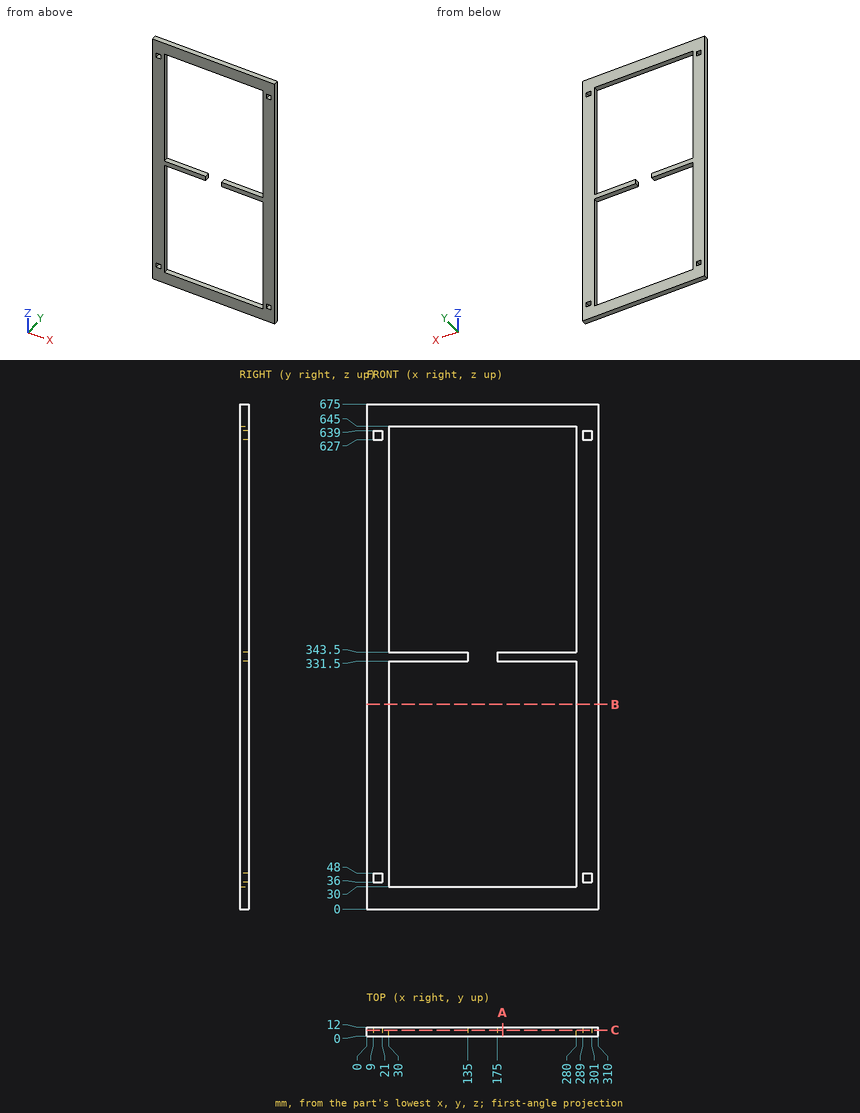
Study the drawing (mm; zero at the part's minimum x, y, z) and answer. Give positions to 0.01 mm unless a question says otherwise; leave off trailing zeros. Loops run counter-clockwise (first coordinate to the right, second up) from the corner with the lowest first, then second, coordinate; pieces in that order, holes last. Notation, with made-up numbers: (55, -9.75) - (110, -9.75) arc R11 cw to (110, -5.75) - close; hole circle Ø2 at (30, 7.25). An arc over 180 degrees is marked (long way). Return JSON: item names as keys, results as strings. Group by question number.
1. Find section C-C (y = 7.75). State how many separate pieces and enclosed holes the cut face has, then the cut area to 3 significant figures.
2. Find section B-B (z = 273.5). Write down the section's boundary in (x, y).
3. Find section A-A (x = 182). Write down the section's boundary in (y, z), then the cut area to 3 significant figures.
4. Straight lines are drawn through the part: line 1 (Z direction, x = 106, y = 11.25); line 2 (X direction, y = 8.5, z = 381); line 3 (Z direction, x = 142.5, y = 4.5). For each, find the intervals that lie inside material, in ascending order. Write a range as [from, to].
Verdict:
{
 "1": {"separate pieces": "1", "enclosed holes": "5", "area": "57,400 mm^2"},
 "2": {"outline": "(0, 0) - (30, 0) - (30, 12) - (0, 12) - close; (280, 0) - (310, 0) - (310, 12) - (280, 12) - close"},
 "3": {"outline": "(0, 0) - (12, 0) - (12, 30) - (0, 30) - close; (0, 331.5) - (12, 331.5) - (12, 343.5) - (0, 343.5) - close; (0, 645) - (12, 645) - (12, 675) - (0, 675) - close", "area": "864 mm^2"},
 "4": {"line 1": "z = [0, 30], [331.5, 343.5], [645, 675]", "line 2": "x = [0, 30], [280, 310]", "line 3": "z = [0, 30], [645, 675]"}
}
